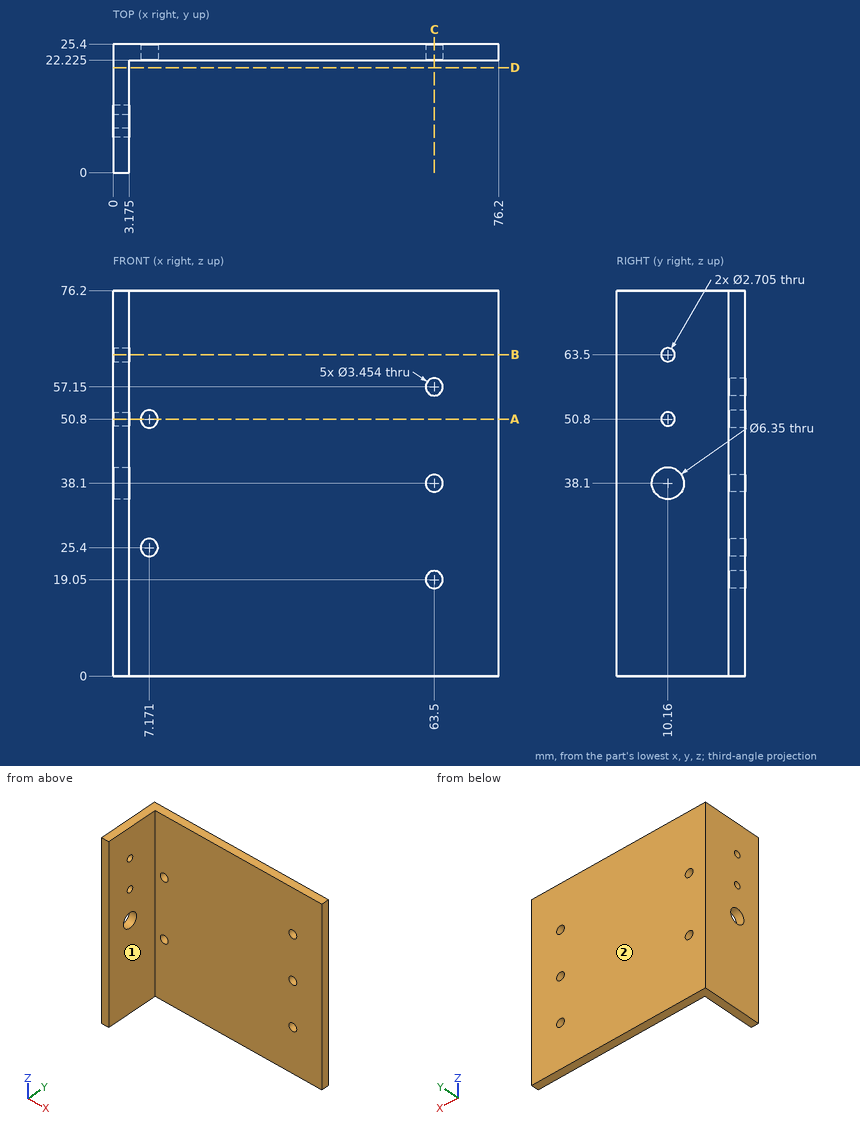
Geometry check sheet. Reference: drawing and pictorial views, mm from the part's lowest x, y, z. A direction names the side the tool comes from. Give positions to 0.01 mm unless a question says otherwise; leave off trailing zeros. Order: outer loops, then holes, each group sorted by start corner. A loop starts at its lowest first (then second) coordinate and runs counter-clockwise, first axis right, second up. Notation, with made-up numbers: M -20,-29.5 L -5,-29.5 A25 cw -5,-2.5 Z; hole C 68,58 d2. An arc over 180 degrees is marked long. Return JSON: item names as keys, results as strings. Group by question number.
1) Scan lines: line 1 (Z direction, x = 63.5, y = 23.15); line 2 (X direction, y = 23.85, z = 50.8) (1 decimal); line 3 (X direction, y = 23.85, z = 38.1). Record each from-to range of solid material in increasing order.
2) Section check B-B on z = 63.5. Record the cut outline in (x, y) (1 decimal), and give its area (3 significant figures).
3) Go/stop test with flat-tipped pins: pin 1 Ø1.5 at (x, z) = (35, 10) entering from -Y (1 decimal); pin 2 Ø3 at (y, z) = (18, 9.5) entering from +X (1 decimal). Record where each tip stops, or that it passes through.
4) Section check C-C on x = 63.5. Record the cut outline in (y, z) (1 decimal).
5) Access from +Z, -Z, +X, -X, +Y, -Y to the whole of each face (thin tool, end or side, straight path). Record for the marked faces 1 and 2.
6) Section check D-D on y = 20.75. Record the cut outline in (x, z) (1 decimal).
7) Section check A-A on z = 50.8. Record the cut outline in (x, y) (1 decimal).
Answer block:
{
 "1": {"line 1": "z = 0 to 17.32, 20.78 to 36.37, 39.83 to 55.42, 58.88 to 76.2", "line 2": "x = 0 to 5.4, 8.9 to 76.2", "line 3": "x = 0 to 61.77, 65.23 to 76.2"},
 "2": {"outline": "M 0,0 L 3.2,0 L 3.2,8.8 L 0,8.8 Z; M 0,11.5 L 3.2,11.5 L 3.2,22.2 L 76.2,22.2 L 76.2,25.4 L 0,25.4 Z", "area": "304 mm^2"},
 "3": {"pin 1": "stops at y = 22.2", "pin 2": "stops at x = 3.2"},
 "4": {"outline": "M 22.2,0 L 25.4,0 L 25.4,17.3 L 22.2,17.3 Z; M 22.2,20.8 L 25.4,20.8 L 25.4,36.4 L 22.2,36.4 Z; M 22.2,39.8 L 25.4,39.8 L 25.4,55.4 L 22.2,55.4 Z; M 22.2,58.9 L 25.4,58.9 L 25.4,76.2 L 22.2,76.2 Z"},
 "5": {"face 1": "+Z, -Z, +X, -Y", "face 2": "+Z, -Z, +X, -X, +Y"},
 "6": {"outline": "M 0,0 L 3.2,0 L 3.2,76.2 L 0,76.2 Z"},
 "7": {"outline": "M 0,0 L 3.2,0 L 3.2,8.8 L 0,8.8 Z; M 0,11.5 L 3.2,11.5 L 3.2,22.2 L 5.4,22.2 L 5.4,25.4 L 0,25.4 Z; M 8.9,22.2 L 76.2,22.2 L 76.2,25.4 L 8.9,25.4 Z"}
}
